```python
from build123d import *

# Parameters (mm, degrees)
SKETCH1_W                                       = 88.9
SKETCH1_H                                       = 88.9
BOSS_EXTRUDE1_DEPTH                             = 3.175
SKETCH3_R                                       = 6.018919743
CUT_EXTRUDE1_DEPTH                              = 4.175
MIRROR2_COPY_1_SKETCH_R                         = 6.018919743
MIRROR2_COPY_1_DEPTH                            = 4.175
SKETCH4_R                                       = 6.35
CUT_EXTRUDE2_DEPTH                              = 4.175
CSK_FOR_M3_FLAT_HEAD_MACHINE_SCREW1_D           = 3.4
CSK_FOR_M3_FLAT_HEAD_MACHINE_SCREW1_CSINK_D     = 6.3
CSK_FOR_M3_FLAT_HEAD_MACHINE_SCREW1_CSINK_ANGLE = 90
CIRPATTERN1_COUNT                               = 6


with BuildPart() as part:
    # Sketch1 → Boss-Extrude1 (new body)
    with BuildSketch(Plane.XY):
        Rectangle(SKETCH1_W, SKETCH1_H)
    extrude(amount=BOSS_EXTRUDE1_DEPTH)

    # Sketch3 → Cut-Extrude1 (cut, through all)
    with BuildSketch(Plane.XY.offset(3.175)):
        with Locations((-31.75, 31.75)):
            Circle(SKETCH3_R)
    cut_extrude1 = extrude(amount=-CUT_EXTRUDE1_DEPTH, mode=Mode.SUBTRACT)

    # Mirror1: Cut-Extrude1 across plane
    add(cut_extrude1.mirror(Plane(origin=(0, 0, 0), x_dir=(0, 0, 1), z_dir=(1, 0, 0))), mode=Mode.SUBTRACT)

    # Mirror2: Cut-Extrude1 across plane
    add(cut_extrude1.mirror(Plane.ZX), mode=Mode.SUBTRACT)

    # Mirror2 copy 1 sketch → Mirror2 copy 1 (cut, through all)
    with BuildSketch(Plane(origin=(0, 0, 3.175), x_dir=(-1, 0, 0), z_dir=(0, 0, 1))):
        with Locations((-31.75, 31.75)):
            Circle(MIRROR2_COPY_1_SKETCH_R)
    extrude(amount=-MIRROR2_COPY_1_DEPTH, mode=Mode.SUBTRACT)

    # Sketch4 → Cut-Extrude2 (cut, through all)
    with BuildSketch(Plane.XY.offset(3.175)):
        Circle(SKETCH4_R)
    extrude(amount=-CUT_EXTRUDE2_DEPTH, mode=Mode.SUBTRACT)

    # CSK for M3 Flat Head Machine Screw1 (through all)
    with Locations(Plane.XY.offset(3.175)):
        with Locations((0, 12.5)):
            csk_for_m3_flat_head_machine_screw1 = CounterSinkHole(CSK_FOR_M3_FLAT_HEAD_MACHINE_SCREW1_D / 2, CSK_FOR_M3_FLAT_HEAD_MACHINE_SCREW1_CSINK_D / 2, counter_sink_angle=CSK_FOR_M3_FLAT_HEAD_MACHINE_SCREW1_CSINK_ANGLE)

    # CirPattern1: CSK for M3 Flat Head Machine Screw1 ×6 about axis
    cirpattern1_axis = Axis((0, 0, 0), (0, 0, 1))
    for i in range(1, CIRPATTERN1_COUNT):
        add(csk_for_m3_flat_head_machine_screw1.rotate(cirpattern1_axis, i * 360 / CIRPATTERN1_COUNT), mode=Mode.SUBTRACT)


solid = part.part
```
Geometry check sheet. Reference: the model listing, model coordinates, mm. Coordinates: 2 decimals unless noted, no trailing zeros. Order: outer loops, then holes, each group sorted by start corner. A loop starts at its lowest first (then second) coordinate and runs counter-clockwise, first axis right, second up.
Q1. Sectioned sample at D-D on z = 2.35. Give the number of separate pieces and of enclosed holes in the cut face, and give its area (3 significant figures).
Reply:
separate pieces: 1
enclosed holes: 11
area: 7,220 mm2
Q2. Sectioned sample at B-B on x = 31.75. Record the cut outline in (y, z) (3 decimals).
Reply:
outline: (-44.45, 0) - (-37.769, 0) - (-37.769, 3.175) - (-44.45, 3.175) - close; (-25.731, 0) - (25.731, 0) - (25.731, 3.175) - (-25.731, 3.175) - close; (37.769, 0) - (44.45, 0) - (44.45, 3.175) - (37.769, 3.175) - close
Q3. Depth check by flat-ended pin: pin 1 Ø4.5 at (x, y) = (0, 12.5) entering from +Z (3 decimals). Enter the tip coordinate at first touch or a pass-through.
Reply:
pin 1: stops at z = 2.275
Q4. Thickness scan on probe 1 along Y at (x, z) = (0, 1.2); probe 2 along Y at (x, z) = (10.5, 2.45); probe 3 along Y at (x, z) = (-5.5, 1.7). Record the ranges inside material, lowest first.
Reply:
probe 1: y = -44.45 to -14.2, -10.8 to -6.35, 6.35 to 10.8, 14.2 to 44.45
probe 2: y = -44.45 to -8.65, -3.85 to 3.85, 8.65 to 44.45
probe 3: y = -44.45 to -3.17, 3.17 to 44.45
Q5. Draft check along Y on faces 1 (the face through (-12.396, -6.901, 0.85)), 2 (the face through (-1, 44.45, 2)), 3 (the face through (9, 1, 3.175)). Enter one of: released by +Y, released by -Y, zero draft, split by the parting line, or undercut.
Reply:
face 1: undercut
face 2: released by +Y
face 3: zero draft
Q6. Sectioned sample at A-A on y = -12.5. Record the cut outline in (x, z) (3 decimals).
Reply:
outline: (-44.45, 0) - (-1.7, 0) - (-1.7, 1.725) - (-3.15, 3.175) - (-44.45, 3.175) - close; (1.7, 0) - (44.45, 0) - (44.45, 3.175) - (3.15, 3.175) - (1.7, 1.725) - close
